Check sheet for the modelled part. Datum: model origin and axes. Units: mm. A direction names the side the tool comes from. Give positions to 0.01 mm unless a question says otherwise; leave off trailing zeros. Write each loop counter-clockwise with the first axis right and the second up, starting at its lowest first coordinate (ties: lowest second). Pieces come first, ordered by that corner, then holes. Notation, with made-up numbers: M 5,62.25 L 33,62.25 A21 cw 33,99.25 Z; hole C -40,62 d4. An arc over 180 degrees is marked long. Write item = value, one per line. Start each with the question number.
1) Set-up check for faces 4 (the face through (92.308, 43.966, 30.521)), 5 (the face through (60.292, 41.308, 5.166)), 6 (the face through (120, 48, 30)): record each of +Z, -Z, +X, -X, +Y, -Y from which the full face is reachable in a straight line by a thin tool's end or side.
2) Gauge pin test, flat end, axial feed: pin 1 (9 mm diameter, centred on y = 40, z = 29.5, fed in from +X). Record the tip position at first contact, or that the pin passes through.
3) Sectioned sample at B-B, the plane x = 101. Record the cut outline in (y, z).
4) Scan lines: L1, parallel to Y at x = 103, z = 30; L2, parallel to Y at x = 117, z = 30; L3, parallel to X at y = 45.5, z = 29. Record each from-to range of solid material in increasing order.
5) Draft check along X on faces 1 (the face through (70, 40, 30)), 2 (the face through (59.855, 23.482, 28.808)), 3 (the face through (59, 0, 20)). Enter one of: pulls with the +X half, pulls with the -X half, needs draft (parallel to the pull), parting line crosses it, or undercut.
6) Sectioned sample at C-C, the plane z = 30. Count the separate pieces of the cut face and the enclosed holes in it, then the cut area to 3 significant figures.
7) Sectioned sample at A-A, the plane x = 25. Record the cut outline in (y, z), then the cut area to 3 significant figures.
from build123d import *

# Parameters (mm, degrees)
SKETCH_1_W          = 120
SKETCH_1_H          = 80
EXTRUDE_1_DEPTH     = 60
CUT_EXTRUDE_1_DEPTH = 157.204993518
SWEEP_2_PROFILE_R   = 6
CUT_EXTRUDE_2_DEPTH = 3.602159411
CUT_EXTRUDE_2_DRAFT = -59
SKETCH_5_R          = 7
CUT_EXTRUDE_3_DEPTH = 6
SKETCH_6_R          = 4
CUT_EXTRUDE_4_DEPTH = 50
SWEEP_4_PROFILE_R   = 5


with BuildPart() as part:
    # 草图1 → 凸台-拉伸1 (new body)
    with BuildSketch(Plane.XY):
        with Locations((60, 40)):
            Rectangle(SKETCH_1_W, SKETCH_1_H)
    extrude(amount=EXTRUDE_1_DEPTH)

    # 草图2 → 切除-拉伸1 (cut, through all)
    with BuildSketch(Plane(origin=(0, 0, 0), x_dir=(0, 0, -1), z_dir=(1, 0, 0))):
        Polygon((-40, 0), (-60, 0), (-60, 28.56287), align=None)
    extrude(amount=CUT_EXTRUDE_1_DEPTH, mode=Mode.SUBTRACT)

    # 切除-扫描2: sweep along a curve in space
    with BuildLine() as sweep_2_path:
        Line((36.683319, 57.441689, 69.112507), (58.926443, 41.066649, 8.000026))
    # 切除-扫描2 profile (on start of the path) → 切除-扫描2 (sweep, cut)
    with BuildSketch(Plane(origin=(36.683319, 57.441689, 69.112507), x_dir=(-0.9396926209151826, 0, -0.34202014297049077), z_dir=(0.3316681247446686, -0.24416888605300846, -0.9112506845605045))):
        Circle(SWEEP_2_PROFILE_R)
    sweep(path=sweep_2_path.line, mode=Mode.SUBTRACT)


with BuildPart() as cut_extrude_2_tool:
    # 草图4 → 切除-拉伸2 (with draft: the straight prism first)
    with BuildSketch(Plane(origin=(0.738557167, -0.543714235, -2.029169141), x_dir=(0.9433961283725703, 0.08584202767282707, 0.3203668073578514), z_dir=(-0.3316681247446686, 0.2441688860530088, 0.9112506845605044))):
        with BuildLine():
            ThreePointArc((61.679165391, 31.596777759), (67.679165393, 37.596777757), (61.679165395, 43.596777759))
            ThreePointArc((61.679165395, 43.596777759), (55.679165393, 37.596777761), (61.679165391, 31.596777759))
        make_face()
    extrude(amount=-CUT_EXTRUDE_2_DEPTH)
    # 切除-拉伸2: the draft: its side faces are tilted about the plane it starts from
    cut_extrude_2_sides = [cut_extrude_2_tool.faces().sort_by_distance(p)[0] for p in [
        (59.523803726, 34.831326418, 7.911705161),
    ]]
    draft(cut_extrude_2_sides, Plane(origin=(0.738557167, -0.543714235, -2.029169141), x_dir=(0.9433961283725703, 0.08584202767282707, 0.3203668073578514), z_dir=(-0.3316681247446686, 0.2441688860530088, 0.9112506845605044)), CUT_EXTRUDE_2_DRAFT)


with BuildPart() as part_1:
    add(part.part)

    # 切除-拉伸2: cut by cut_extrude_2_tool
    add(cut_extrude_2_tool.part, mode=Mode.SUBTRACT)

    # 草图5 → 切除-拉伸3 (cut)
    with BuildSketch(Plane(origin=(120, 0, 0), x_dir=(0, 0, -1), z_dir=(1, 0, 0))):
        with Locations((-30, 40)):
            Circle(SKETCH_5_R)
    extrude(amount=-CUT_EXTRUDE_3_DEPTH, mode=Mode.SUBTRACT)

    # 草图6 → 切除-拉伸4 (cut)
    with BuildSketch(Plane(origin=(120, 0, 0), x_dir=(0, 0, -1), z_dir=(1, 0, 0))):
        with Locations((-30, 40)):
            Circle(SKETCH_6_R)
    extrude(amount=-CUT_EXTRUDE_4_DEPTH, mode=Mode.SUBTRACT)

    # 切除-扫描4: sweep along a curve in space
    with BuildLine() as sweep_4_path:
        Line((57.9403, 8.545716, 58.19152), (57.9403, 41.792672, 10.709946))
    # 切除-扫描4 profile (on start of the path) → 切除-扫描4 (sweep, cut)
    with BuildSketch(Plane(origin=(57.9403, 8.545716, 58.19152), x_dir=(0, -0.8191520446202117, -0.573576435878015), z_dir=(0, 0.573576435878015, -0.8191520446202117))):
        Circle(SWEEP_4_PROFILE_R)
    sweep(path=sweep_4_path.line, mode=Mode.SUBTRACT)


solid = part_1.part
Data:
q1.face_4 = +X
q1.face_5 = none
q1.face_6 = +Z, -Z, +X, +Y, -Y
q2.pin_1 = 114
q3.outline = M 0,0 L 80,0 L 80,60 L 28.56,60 L 0,40 Z; hole C 40,30 d8
q4.L1 = 0 to 36, 44 to 80
q4.L2 = 0 to 33, 47 to 80
q4.L3 = 0 to 45.15, 57.63 to 114
q5.face_1 = pulls with the +X half
q5.face_2 = undercut
q5.face_3 = needs draft
q6.separate_pieces = 1
q6.enclosed_holes = 2
q6.area = 8,940 mm2
q7.outline = M 0,0 L 80,0 L 80,60 L 28.56,60 L 0,40 Z
q7.area = 4,510 mm2
